Autodesk Inventor part; units mm, degrees
ref_plane "YZ Plane" through (0, 0, 0) normal (1, 0, 0) x (0, 1, 0)
ref_plane "XZ Plane" through (0, 0, 0) normal (0, 1, 0) x (-1, 0, 0)
ref_plane "XY Plane" through (0, 0, 0) normal (0, 0, 1) x (1, 0, 0)
sketch "Sketch1" plane through (0, 0, 0) normal (0, 0, 1) x (1, 0, 0)
  circle A0 centre (44.9, 4.9) radius 1.45 construction
  circle A1 centre (4.9, 4.9) radius 1.45 construction
  line L0 (2, 2) -> (2, 41.8) construction
  line L1 (47.8, 2) -> (2, 2) construction
  line L2 (47.8, 41.8) -> (47.8, 2) construction
  line L3 (41.8, 41.8) -> (47.8, 41.8) construction
  line L4 (41.8, 8) -> (41.8, 41.8) construction
  line L5 (8, 8) -> (41.8, 8) construction
  line L6 (8, 8) -> (8, 41.8) construction
  line L7 (2, 41.8) -> (8, 41.8) construction
  circle A2 centre (44.9, 44.9) radius 1.4 construction
  circle A3 centre (4.9, 44.9) radius 1.4 construction
  line L8 (2, 47.8) -> (47.8, 47.8) construction
  line L9 (2, 41.8) -> (2, 47.8) construction
  line L10 (47.8, 41.8) -> (2, 41.8) construction
  line L11 (47.8, 41.8) -> (47.8, 47.8) construction
  circle A4 centre (25.6838, 25.4066) radius 13.6 construction
  line L12 (44.1319, 49.8) -> (5.6681, 49.8) construction
  arc A5 (49.8, 47.8) -> (47.8, 49.8) centre (47.8, 47.8) ccw construction
  line L13 (49.8, 41.8) -> (49.8, 47.8) construction
  arc A6 (2, 49.8) -> (0, 47.8) centre (2, 47.8) ccw construction
  arc A7 (0, 2) -> (2, 0) centre (2, 2) ccw construction
  arc A8 (47.8, 0) -> (49.8, 2) centre (47.8, 2) ccw construction
  line L14 (49.8, 0) -> (-62.2, 0)
  line L15 (-62.2, 0) -> (-62.2, 49.8)
  line L16 (-62.2, 49.8) -> (49.8, 49.8)
  line L17 (49.8, 49.8) -> (49.8, 0)
  line L18 (8, 3.7577) -> (41.8, 3.7577) construction
  line L19 (41.8, 0) -> (41.8, 3.7577) construction
  line L20 (8, 0) -> (41.8, 0) construction
  line L21 (8, 0) -> (8, 3.7577) construction
  line L22 (46.1838, 8) -> (46.1838, 41.8) construction
  line L23 (49.8, 41.8) -> (46.1838, 41.8) construction
  line L24 (49.8, 8) -> (49.8, 41.8) construction
  line L25 (46.1838, 8) -> (49.8, 8) construction
  line L26 (3.6162, 41.8) -> (3.6162, 8) construction
  line L27 (0, 8) -> (3.6162, 8) construction
  line L28 (0, 8) -> (0, 41.8) construction
  line L29 (3.6162, 41.8) -> (0, 41.8) construction
  circle A9 centre (24.9, 24.9) radius 15
  arc A10 (42.3945, 24.4616) -> (22.4616, 42.2293) centre (24.9, 24.9) ccw construction
  arc A11 (22.5619, 16.1033) -> (42.3945, 24.4616) centre (29.0002, 28.5351) ccw construction
  line L30 (22.5619, 16.1033) -> (22.3031, 15.1374) construction
  arc A12 (22.3031, 15.1374) -> (41.5232, 19.4302) centre (29.3361, 28.8218) ccw construction
  arc A13 (15.3425, 10.2404) -> (41.5232, 19.4302) centre (24.9, 24.9) ccw construction
  arc A14 (18.2047, 31.6263) -> (15.3425, 10.2404) centre (25.6173, 19.7498) ccw construction
  line L31 (18.2047, 31.6263) -> (17.4976, 32.3335) construction
  arc A15 (17.4976, 32.3335) -> (11.1478, 14.0775) centre (25.6302, 19.2725) ccw construction
  arc A16 (16.2809, 40.1303) -> (11.1478, 14.0775) centre (24.9, 24.9) ccw construction
  arc A17 (34.0602, 27.4798) -> (16.2809, 40.1303) centre (20.0844, 26.6568) ccw construction
  line L32 (34.0602, 27.4798) -> (35.0261, 27.7386) construction
  arc A18 (35.0261, 27.7386) -> (22.4616, 42.2293) centre (19.6533, 27.1018) ccw construction
  line L33 (3.6577, 41.7) -> (8.1, 46.1423) construction
  line L34 (0, 41.7) -> (3.6577, 41.7) construction
  line L35 (0, 8.1) -> (0, 41.7) construction
  line L36 (3.6577, 8.1) -> (0, 8.1) construction
  line L37 (8.1, 3.6577) -> (3.6577, 8.1) construction
  line L38 (8.1, 0) -> (8.1, 3.6577) construction
  line L39 (41.7, 0) -> (8.1, 0) construction
  line L40 (41.7, 3.6577) -> (41.7, 0) construction
  line L41 (46.1423, 8.1) -> (41.7, 3.6577) construction
  line L42 (49.8, 8.1) -> (46.1423, 8.1) construction
  line L43 (49.8, 41.7) -> (49.8, 8.1) construction
  line L44 (46.1423, 41.7) -> (49.8, 41.7) construction
  line L45 (41.7, 46.1423) -> (46.1423, 41.7) construction
  line L46 (41.7, 49.8) -> (41.7, 46.1423) construction
  line L47 (8.1, 49.8) -> (41.7, 49.8) construction
  line L48 (8.1, 46.1423) -> (8.1, 49.8) construction
  circle A19 centre (24.9, 24.9) radius 16.9 construction
  point P0 (0, 0)
  dimension "d0" = 30
  dimension "d4" = 112
extrude "Extrusion1" add sketch "Sketch1" along normal blind 11.4
fillet "Fillet1" radius 2 4 edges at (49.8, 49.8, 5.7) (-62.2, 49.8, 5.7) (49.8, 0, 5.7) (-62.2, 0, 5.7)
sketch "Sketch2" plane through (0, 0, 0) normal (0, 0, -1) x (-1, 0, 0)
  line L0 (-41.8, 8) -> (-41.8, 41.8) construction
  line L1 (-8, 8) -> (-41.8, 8) construction
  line L2 (-8, 8) -> (-8, 41.8) construction
  line L3 (-47.8, 41.8) -> (-2, 41.8) construction
  circle A0 centre (-24.9, 24.9) radius 15 construction
  arc A1 (60.2, 0) -> (62.2, 2) centre (60.2, 2) ccw construction
  line L4 (62.2, 2) -> (62.2, 47.8) construction
  arc A2 (62.2, 47.8) -> (60.2, 49.8) centre (60.2, 47.8) ccw construction
  line L5 (60.2, 49.8) -> (-47.8, 49.8) construction
  arc A3 (-47.8, 49.8) -> (-49.8, 47.8) centre (-47.8, 47.8) ccw construction
  line L6 (-49.8, 47.8) -> (-49.8, 2) construction
  arc A4 (-49.8, 2) -> (-47.8, 0) centre (-47.8, 2) ccw construction
  line L7 (-47.8, 0) -> (60.2, 0) construction
  line L8 (-41.8, 41.8) -> (-8, 41.8)
  line L9 (-8, 41.8) -> (-8, 8)
  line L10 (-8, 8) -> (-41.8, 8)
  line L11 (-41.8, 8) -> (-41.8, 41.8)
  line L12 (-9, 40.8) -> (-40.8, 40.8)
  line L13 (-40.8, 40.8) -> (-40.8, 9)
  line L14 (-40.8, 9) -> (-9, 9)
  line L15 (-9, 9) -> (-9, 40.8)
  point P0 (0, 0)
  dimension "d6" = 0
  dimension "d7" = 0
  dimension "d8" = 0
  dimension "d9" = 0
  dimension "d10" = 1
extrude "Extrusion2" add sketch "Sketch2" along normal blind 3.66
sketch "Sketch3" plane through (8, 8, 0) normal (0, -1, 0) x (1, 0, 0)
  line L0 (0, 0) -> (33.8, 0) construction
  line L1 (0, 0) -> (0, -3.66) construction
  line L2 (33.8, -3.66) -> (0, -3.66) construction
  line L3 (33.8, 0) -> (33.8, -3.66) construction
  line L4 (33.5, -3.7577) -> (33.5, -8) construction
  line L5 (-0.3, -8) -> (33.5, -8) construction
  line L6 (-0.3, -3.7577) -> (-0.3, -8) construction
  line L7 (33.5, -3.7577) -> (-0.3, -3.7577) construction
  line L8 (33.5, 0) -> (33.5, -3.6162) construction
  line L9 (-0.3, -3.6162) -> (-0.3, 0) construction
  line L10 (33.8, 0) -> (33.8, -3.66) construction
  line L11 (33.8, 0) -> (33.8, -3.66) construction
  line L12 (33.5, -8) -> (33.5, -3.7577) construction
  line L13 (33.5, -3.7577) -> (-0.3, -3.7577) construction
  line L14 (-0.3, -3.7577) -> (-0.3, -8) construction
  line L15 (-0.3, -8) -> (-4.6838, -8) construction
  line L16 (-2.886, -6.2022) -> (-4.6838, -8) construction
  arc A0 (-2.886, -6.2022) -> (-2.0978, -5.414) centre (-3.4, -4.9) ccw construction
  line L17 (-0.3, -3.6162) -> (-2.0978, -5.414) construction
  line L18 (-0.3, -3.6162) -> (-0.3, 0) construction
  line L19 (-0.3, 0) -> (33.5, 0) construction
  line L20 (33.5, 0) -> (33.5, -3.6162) construction
  line L21 (35.2978, -5.414) -> (33.5, -3.6162) construction
  arc A1 (35.2978, -5.414) -> (36.086, -6.2022) centre (36.6, -4.9) ccw construction
  line L22 (37.8838, -8) -> (36.086, -6.2022) construction
  line L23 (37.8838, -8) -> (33.5, -8) construction
  line L24 (0, -3.66) -> (33.8, -3.66)
  line L25 (0, -3.66) -> (-4.34, -8)
  line L26 (-4.34, -8) -> (-2.2187, -8)
  line L27 (-2.2187, -8) -> (2.1213, -3.66)
  line L28 (16.6, -3.7577) -> (16.6, -8) construction
  line L29 (2.1213, -3.66) -> (0, -3.66)
  line L30 (1, -3.66) -> (32.8, -3.66)
  line L31 (33.5, -3.7577) -> (33.5, -8) construction
  line L32 (33.5, -3.7577) -> (33.5, -8) construction
  line L33 (33.5, -8) -> (37.8838, -8) construction
  line L34 (36.086, -6.2022) -> (37.8838, -8) construction
  arc A2 (35.2978, -5.414) -> (36.086, -6.2022) centre (36.6, -4.9) ccw construction
  line L35 (33.5, -3.6162) -> (35.2978, -5.414) construction
  line L36 (33.2, -3.66) -> (37.54, -8)
  line L37 (37.54, -8) -> (35.4187, -8)
  line L38 (35.4187, -8) -> (31.0787, -3.66)
  line L39 (31.0787, -3.66) -> (33.2, -3.66)
  point P0 (-8, 0)
  point P1 (32.2, -3.66)
  dimension "d13" = 1.5
extrude "Extrusion3" add sketch "Sketch3" against normal up to surface (33.8 mm away)
sketch "Sketch4" plane through (0, 0, 0) normal (0, 0, -1) x (-1, 0, 0)
  arc A0 (60.2, 0) -> (62.2, 2) centre (60.2, 2) ccw construction
  line L0 (62.2, 2) -> (62.2, 47.8) construction
  arc A1 (62.2, 47.8) -> (60.2, 49.8) centre (60.2, 47.8) ccw construction
  line L1 (60.2, 49.8) -> (-47.8, 49.8) construction
  arc A2 (-47.8, 49.8) -> (-49.8, 47.8) centre (-47.8, 47.8) ccw construction
  line L2 (-49.8, 47.8) -> (-49.8, 2) construction
  arc A3 (-49.8, 2) -> (-47.8, 0) centre (-47.8, 2) ccw construction
  line L3 (-47.8, 0) -> (60.2, 0) construction
  line L4 (-8, 41.8) -> (-8, 8) construction
  line L5 (-8, 8) -> (-41.8, 8) construction
  line L6 (-41.8, 8) -> (-41.8, 41.8) construction
  line L7 (-41.8, 41.8) -> (-8, 41.8) construction
  line L8 (-4.8, 44.8) -> (57.2, 44.8)
  line L9 (57.2, 44.8) -> (57.2, 5)
  line L10 (57.2, 5) -> (-4.8, 5)
  line L11 (-4.8, 5) -> (-4.8, 44.8)
  point P0 (0, 0)
  dimension "d16" = 45
  dimension "d17" = 5
  dimension "d18" = 5
  dimension "d19" = 5
extrude "Extrusion4" cut sketch "Sketch4" against normal through all
fillet "Fillet2" radius 2 4 edges at (4.8, 5, 5.7) (-57.2, 5, 5.7) (-57.2, 44.8, 5.7) (4.8, 44.8, 5.7)
equation "\"d18\" = d17"
equation "\"d19\" = d17"
properties part number "30_Smartphone_Holder_v3"
Check sheet for the modelled part. Datum: model origin and axes. Units: mm. A direction names the side the tool comes from. Coordinates: 2 decimals unless noted, no trailing zeros. Write each loop counter-clockwise with the first axis right and the second up, starting at its lowest first coordinate (ties: lowest second). Pieces come first, ordered by that corner, then holes.
Item 1: Cross-section at A-A on y = 24.9. Record the boundary of the cut face in (x, z), then the cut area to 3 significant figures.
Numbers:
outline: (-62.2, 0) - (-57.2, 0) - (-57.2, 11.4) - (-62.2, 11.4) - close; (3.66, -8) - (5.78, -8) - (10.12, -3.66) - (9, -3.66) - (9, 0) - (9.9, 0) - (9.9, 11.4) - (4.8, 11.4) - (4.8, 0) - (8, 0) - (8, -3.66) - close; (39.08, -3.66) - (43.42, -8) - (45.54, -8) - (41.2, -3.66) - (41.8, -3.66) - (41.8, 0) - (49.8, 0) - (49.8, 11.4) - (39.9, 11.4) - (39.9, 0) - (40.8, 0) - (40.8, -3.66) - close
area: 254 mm2
Item 2: Depth check by flat-ended pin: pin 1 Ø2 at (x, z) = (28.5, -1.5) entering from -Y; pin 2 Ø0.8 at (x, y) = (29, 8.5) entering from -Z; pin 3 Ø1.8 at (y, z) = (23, -2) entering from -X. Enter the tip coordinate at first touch or a pass-through.
Numbers:
pin 1: stops at y = 8
pin 2: stops at z = -3.66
pin 3: stops at x = 8
Item 3: Cross-section at D-D on z = -2.25. Record the boundary of the cut face in (x, y), then the cut area to 3 significant figures.
Numbers:
outline: (8, 8) - (41.8, 8) - (41.8, 41.8) - (8, 41.8) - close; hole (9, 9) - (40.8, 9) - (40.8, 40.8) - (9, 40.8) - close
area: 131 mm2
Item 4: Cross-section at C-C on z = 2.25. Record the boundary of the cut face in (x, y), then the cut area to 3 significant figures.
Numbers:
outline: (-62.2, 2) arc R2 ccw to (-60.2, 0) - (47.8, 0) arc R2 ccw to (49.8, 2) - (49.8, 47.8) arc R2 ccw to (47.8, 49.8) - (-60.2, 49.8) arc R2 ccw to (-62.2, 47.8) - close; hole (-57.2, 7) arc R2 ccw to (-55.2, 5) - (2.8, 5) arc R2 ccw to (4.8, 7) - (4.8, 42.8) arc R2 ccw to (2.8, 44.8) - (-55.2, 44.8) arc R2 ccw to (-57.2, 42.8) - close; hole circle Ø30 at (24.9, 24.9)
area: 2,400 mm2
Item 5: Mould release check, pull along Z, two halves, no side actions. Record for faces 4 (the face through (22.947, 10.028, 5.62)), 5 (the face through (8, 25, -2)), 6 (the face through (7.92, 24.66, -5.86)), 7 (the face through (5, 25, 11.4)): released by +Z, released by -Z, zero draft, split by the parting line, or undercut.
Numbers:
face 4: zero draft
face 5: undercut
face 6: released by -Z
face 7: released by +Z
Item 6: Cross-section at B-B on x = 24.9. Record the boundary of the cut face in (y, z), then the cut area to 3 significant figures.
Numbers:
outline: (0, 0) - (8, 0) - (8, -3.66) - (9, -3.66) - (9, 0) - (9.9, 0) - (9.9, 11.4) - (0, 11.4) - close; (39.9, 0) - (40.8, 0) - (40.8, -3.66) - (41.8, -3.66) - (41.8, 0) - (49.8, 0) - (49.8, 11.4) - (39.9, 11.4) - close
area: 233 mm2
Item 7: Access from +Z, -Z, +X, -X, +Y, -Y to the whole of each face (thin tool, end or side, straight path). Record for faces 1 (the face through (24, 8, -2)), 2 (the face through (25, 41.8, -2)), 3 (the face through (-27, 5, 6)).
Numbers:
face 1: -Z, +X, -X, -Y
face 2: -Z, +X, -X, +Y
face 3: +Z, -Z
Item 8: Scan lines: probe 1 along Y at (x, z) = (-50.5, 8.75); probe 2 along Y at (x, z) = (34.5, -1.75); probe 3 along X at (y, z) = (7, 0.5). Record each from-to range of solid material in increasing order.
Numbers:
probe 1: y = 0 to 5, 44.8 to 49.8
probe 2: y = 8 to 9, 40.8 to 41.8
probe 3: x = -62.2 to -57.2, 4.8 to 49.8
